Could you check a few things on this drawing? It's one solid part, dimensions in mm from its lowest x, y, z. Give positions to 0.01 mm unless a question says otherwise; leave off trailing zeros. Write each loop counter-clockwise with the first axis right and the second up, starting at its lowest first coordinate (ties: lowest second). Pieces come first, ordered by that corner, then holes. Notation, with made-up numbers: M 77,0 L 84,0 A29 cw 84,26 Z; hole C 85.5,-34.75 d9. An arc over 180 degrees is marked long. Answer as CSV lines item,"result". Start each with the question number.
Q1. Suppose I cut it at D-D (y = 8.5). Write out the boundary of the cut face in (x, z), then the cut area to 3 significant figures.
Q2. Suppose I cut it at A-A (y = 27). Write out the boundary of the cut face in (x, z), then the cut area to 3 significant figures.
Q3. Thinking about a two-plate mould opening in X: for the marked faces 1, 2 and 3, which applies, +X half, -X half, draft (parallel to the pull), parting line (faces both ways), or undercut?
Q4. Suppose I cut it at C-C (z = 7.25). Write out the boundary of the cut face in (x, y), then the cut area to 3 significant figures.
Q5. If I drill on line 1 along Y through (x, z) = (27, 5.75); line 2 along Z through (x, y) = (7, 21); line 3 along X through (y, z) = (30.5, 5.5), over which ranges is the centre line in solid material (lowest first)?
Q6. For pin 1 (10 mm diameter, centred on y = 24, z = 2.5, fed in from +X); pin 2 (2 mm diameter, centred on y = 30.5, z = 6, fed in from -X); pin 3 (3 mm diameter, centred on x = 18, y = 44, fed in from -Z), each with a flat end and sliding along its axis, tell me the tip position at first contact or that it passes through.
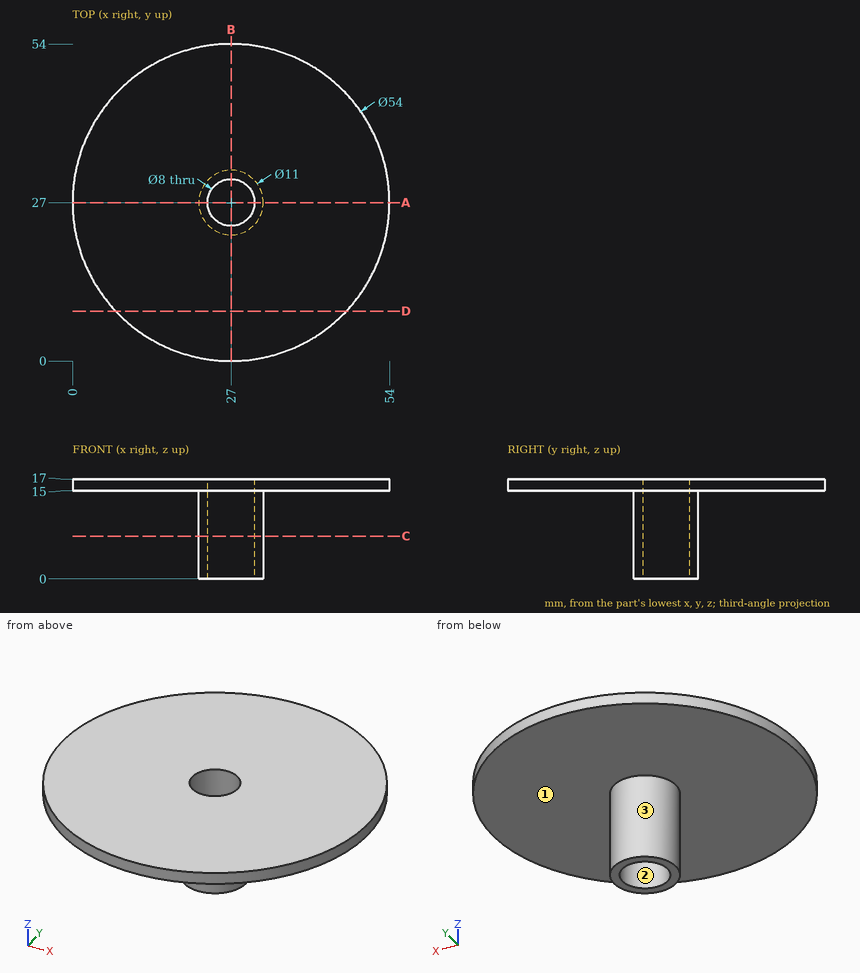
Resolved:
1,outline,"M 7.33,15 L 46.67,15 L 46.67,17 L 7.33,17 Z"
1,area,"78.7 mm^2"
2,outline,"M 0,15 L 21.5,15 L 21.5,0 L 23,0 L 23,17 L 0,17 Z; M 31,0 L 32.5,0 L 32.5,15 L 54,15 L 54,17 L 31,17 Z"
2,area,"137 mm^2"
3,face 1,"draft"
3,face 2,"undercut"
3,face 3,"parting line"
4,outline,"C 27,27 d11; hole C 27,27 d8"
4,area,"44.8 mm^2"
5,line 1,"21.5 to 23, 31 to 32.5"
5,line 2,"15 to 17"
5,line 3,"22.76 to 25.06, 28.94 to 31.24"
6,pin 1,"x = 32.5"
6,pin 2,"x = 22.1"
6,pin 3,"z = 15"
